```python
from build123d import *

# Parameters (mm, degrees)
EXTRUDE_1_DEPTH = 6
CHAMFER_1_SIZE  = 2


with BuildPart() as part:
    # Эскиз1 → Бобышка-Вытянуть1 (new body)
    with BuildSketch(Plane(origin=(0, 0, 0), x_dir=(1, 0, 0), z_dir=(0, 1, 0))):
        Polygon((-2.444490443, 0), (-18.055509557, 0), (-20.5, 7.510567106), (-20.5, 38.754932475), (-18.055509557, 52), (-2.444490443, 52), (0, 38.754932475), (0, 7.510567106), align=None)
    extrude(amount=EXTRUDE_1_DEPTH)

    # Фаска1
    chamfer_1_edges = [part.edges().sort_by_distance(p)[0] for p in [
        (-19.277754779, 6, -3.755283553),
        (-10.25, 6, 0),
        (-1.222245221, 6, -3.755283553),
        (0, 6, -23.13274979),
        (-1.222245221, 6, -45.377466237),
        (-10.25, 6, -52),
        (-20.5, 6, -23.13274979),
    ]]
    chamfer(chamfer_1_edges, length=CHAMFER_1_SIZE)


solid = part.part
```
CAD build for the part. Positions are in the model's coordinates, mm. Round coordinates to 2 decimals unless told otherwise and drop trailing zeros. Order: outer loops, then holes, each group sorted by start corner. A loop starts at its lowest first (then second) coordinate and runs counter-clockwise, first axis right, second up. Notation, with made-up numbers: (14, 18) -> (21, 18) arc R12 ccw to (21, 35) -> close; hole circle Ø1 at (-2.75, 59). An arc over 180 degrees is marked (long way). One line per question, with ' | ' between items.
Q1. Slice it at C-C (y = 4.75). Write the cut outline in (x, z), then the cut area to 3 significant figures.
Completed:
outline: (-19.75, -42.82) -> (-18.19, -51.25) -> (-3.07, -51.25) -> (-0.75, -38.69) -> (-0.75, -7.63) -> (-2.99, -0.75) -> (-17.51, -0.75) -> (-19.75, -7.63) -> close | area: 923 mm^2
Q2. Slice it at B-B (z = -35.5). Write the cut outline in (x, y), then the cut area to 3 significant figures.
Completed:
outline: (-20.5, 0) -> (0, 0) -> (0, 4) -> (-2, 6) -> (-18.5, 6) -> (-20.5, 4) -> close | area: 119 mm^2
Q3. Slice it at D-D (z = -46). Write the cut outline in (x, y), then the cut area to 3 significant figures.
Completed:
outline: (-19.16, 0) -> (-1.34, 0) -> (-1.34, 4) -> (-3.37, 6) -> (-18.5, 6) -> (-19.16, 5.34) -> close | area: 105 mm^2
Q4. Slice it at A-A (y = 2.25). Write the cut outline in (x, z), then the cut area to 3 significant figures.
Completed:
outline: (-20.5, -38.75) -> (-18.06, -52) -> (-2.44, -52) -> (0, -38.75) -> (0, -7.51) -> (-2.44, 0) -> (-18.06, 0) -> (-20.5, -7.51) -> close | area: 1,020 mm^2
Q5. Drop a flat-ended pin along its axis: pin 1 (3 mm diameter, centred on x = -11, z = -11.5, fed in from -Y). Give the stop position or say it passes through.
Completed:
pin 1: stops at y = 0
Q6. Probe probe 1 along X at (y, z) = (5.75, -44); probe 2 along Z at (x, y) = (-15, 4.75); probe 3 along X at (y, z) = (2.5, -45). List the from-to ranges inside material, lowest first.
Completed:
probe 1: x = -18.75 to -2.75 | probe 2: z = -51.25 to -0.75 | probe 3: x = -19.35 to -1.15
